```python
from build123d import *

# Parameters (mm, degrees)
SKETCH1_W               = 8
SKETCH1_H               = 8
BOSS_EXTRUDE1_DEPTH     = 8
SKETCH2_W               = 4
SKETCH2_H               = 4
BOSS_EXTRUDE2_DEPTH     = 5.5
SKETCH3_R               = 0.4
BOSS_EXTRUDE3_DEPTH     = 3.5
SKETCH4_W               = 1
SKETCH4_H               = 4
CUT_EXTRUDE1_DEPTH      = 3
CUT_EXTRUDE2_DEPTH      = 15.637281168
CUT_EXTRUDE2_DEPTH_BACK = 15.637281168
SKETCH5_W               = 0.5
SKETCH5_H               = 3


with BuildPart() as part:
    # Sketch1 → Boss-Extrude1 (new body)
    with BuildSketch(Plane(origin=(0, 0, 0), x_dir=(1, 0, 0), z_dir=(0, 1, 0))):
        Rectangle(SKETCH1_W, SKETCH1_H)
    extrude(amount=BOSS_EXTRUDE1_DEPTH)

    # Sketch2 → Boss-Extrude2 (add)
    with BuildSketch(Plane(origin=(0, 8, 0), x_dir=(1, 0, 0), z_dir=(0, 1, 0))):
        Rectangle(SKETCH2_W, SKETCH2_H)
    extrude(amount=BOSS_EXTRUDE2_DEPTH)

    # Sketch3 → Boss-Extrude3 (add)
    with BuildSketch(Plane.XZ):
        with Locations(Location((0, 3, 0), (0, 0, 90))):
            Circle(SKETCH3_R)
        with Locations(Location((-2.5, 3, 0), (0, 0, 90))):
            Circle(SKETCH3_R)
        with Locations(Location((2.5, 3, 0), (0, 0, 90))):
            Circle(SKETCH3_R)
        with Locations(Location((2.5, -3, 0), (0, 0, 90))):
            Circle(SKETCH3_R)
        with Locations(Location((-2.5, -3, 0), (0, 0, 90))):
            Circle(SKETCH3_R)
        with Locations(Location((0, -3, 0), (0, 0, 90))):
            Circle(SKETCH3_R)
    extrude(amount=BOSS_EXTRUDE3_DEPTH)

    # Sketch4 → Cut-Extrude1 (cut)
    with BuildSketch(Plane(origin=(0, 13.5, 0), x_dir=(1, 0, 0), z_dir=(0, 1, 0))):
        with Locations((-1.5, 0)):
            Rectangle(SKETCH4_W, SKETCH4_H)
        with Locations((1.5, 0)):
            Rectangle(SKETCH4_W, SKETCH4_H)
    extrude(amount=-CUT_EXTRUDE1_DEPTH, mode=Mode.SUBTRACT)

    # Sketch5 → Cut-Extrude2 (cut, two sides: drawn at the far end of the back side and taken through both)
    with BuildSketch(Plane(origin=(0, 0, 0), x_dir=(0, 0, -1), z_dir=(1, 0, 0)).offset(-CUT_EXTRUDE2_DEPTH_BACK)):
        with Locations((-1.75, 12)):
            Rectangle(SKETCH5_W, SKETCH5_H)
        with Locations((1.75, 12)):
            Rectangle(SKETCH5_W, SKETCH5_H)
    extrude(amount=CUT_EXTRUDE2_DEPTH + CUT_EXTRUDE2_DEPTH_BACK, mode=Mode.SUBTRACT)


solid = part.part
```
Input: part model. Units: mm. Frame: model coordinates. A direction names the side the tool comes from. Coordinates: 2 decimals unless noted, no trailing zeros. Write each loop counter-clockwise with the first axis right and the second up, starting at its lowest first coordinate (ties: lowest second). Pieces come first, ordered by that corner, then holes. Notation, with made-up numbers: (-28, 15) - (-10, 15) arc R13 ccw to (-10, 31) - close; hole circle Ø4 at (34.5, 14). An arc over 180 degrees is marked (long way). Put each result on its own line as item: value. Start each with the question number.
1) Reachability of faces 1 (the face through (0, 12, -1.5)), 2 (the face through (0, 9, 2)), 3 (the face through (-1, 12, 0)), 4 (the face through (2, 9, 0)) from +Z, -Z, +X, -X, +Y, -Y: full face, straight path, thin tool, end or side. Return the list, or none.
2) Cut plane A-A (y = -1.5). Return the cut outline in (x, z), plus the area to 3 significant figures.
3) Contact query for flat-ended pins moving along their axis: pin 1 (1.2 mm diameter, centred on x = 1, y = 9.5, fed in from -Z); pin 2 (1.5 mm diameter, centred on x = -0.5, z = 0, fed in from -Y); pin 3 (1.6 mm diameter, centred on x = 0.5, y = 12, fed in from -Z); pin 4 (3 mm diameter, centred on x = 3, z = -2.5, fed in from -Y). Output: stop coordinate, or through.
4) Ray query, L1, parallel to Y at x = 2.75, z = 0.25; L2, parallel to Y at x = 1.25, z = -1.75; L3, parallel to Z at x = 0.25, y = 10. Return the intervals inside material, ascending.
5) Cut plane D-D (y = 11.25). Return the cut outline in (x, z).
6) Mould query, pull axis Z, two halves, no side actions, for faces 5 (the face through (0, 0, 0)), 6 (the face through (0, 12, 1.5)), 7 (the face through (-1.4, 10.5, 0)). Classes: pulls with the +Z half, pulls with the -Z half, needs draft (parallel to the pull), parting line crosses it, or undercut.
7) Cut plane C-C (z = 3). Return the cut outline in (x, y).
8) Cut plane B-B (x = 2.5). Return the cut outline in (y, z).
Resolved:
1. face 1: -Z, +X, -X, +Y
1. face 2: +Z, +X, -X, +Y
1. face 3: +Z, -Z, -X, +Y
1. face 4: +Z, -Z, +X, +Y
2. outline: circle Ø0.8 at (-2.5, -3); circle Ø0.8 at (-2.5, 3); circle Ø0.8 at (0, -3); circle Ø0.8 at (0, 3); circle Ø0.8 at (2.5, -3); circle Ø0.8 at (2.5, 3)
2. area: 3.02 mm2
3. pin 1: stops at z = -2
3. pin 2: stops at y = 0
3. pin 3: stops at z = -1.5
3. pin 4: stops at y = -3.5
4. L1: y = 0 to 8
4. L2: y = 0 to 10.5
4. L3: z = -2 to 2
5. outline: (-1, -1.5) - (1, -1.5) - (1, 1.5) - (-1, 1.5) - close
6. face 5: undercut
6. face 6: pulls with the +Z half
6. face 7: needs draft
7. outline: (-4, 0) - (-2.9, 0) - (-2.9, -3.5) - (-2.1, -3.5) - (-2.1, 0) - (-0.4, 0) - (-0.4, -3.5) - (0.4, -3.5) - (0.4, 0) - (2.1, 0) - (2.1, -3.5) - (2.9, -3.5) - (2.9, 0) - (4, 0) - (4, 8) - (-4, 8) - close
8. outline: (-3.5, -3.4) - (0, -3.4) - (0, -4) - (8, -4) - (8, 4) - (0, 4) - (0, 3.4) - (-3.5, 3.4) - (-3.5, 2.6) - (0, 2.6) - (0, -2.6) - (-3.5, -2.6) - close
